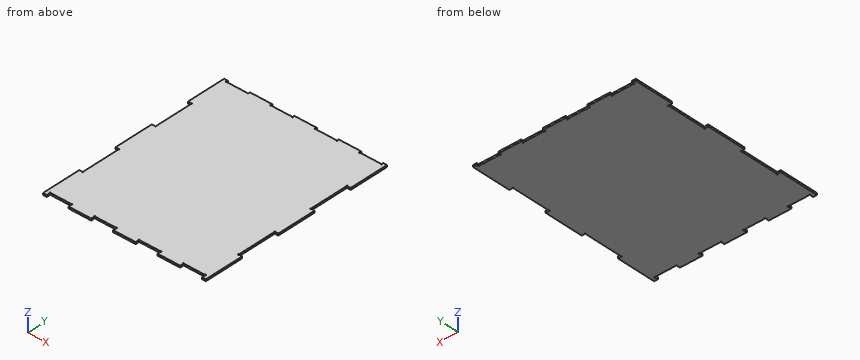
Autodesk Inventor part; units mm, degrees
ref_plane "YZ Plane" through (0, 0, 0) normal (1, 0, 0) x (0, 1, 0)
ref_plane "XZ Plane" through (0, 0, 0) normal (0, 1, 0) x (-1, 0, 0)
ref_plane "XY Plane" through (0, 0, 0) normal (0, 0, 1) x (1, 0, 0)
sketch "Esboço1" plane through (0, 0, 0) normal (0, 0, 1) x (1, 0, 0)
  line L0 (-173, 210) -> (173, 210)
  line L1 (173, 210) -> (173, -210)
  line L2 (173, -210) -> (-173, -210)
  line L3 (-173, -210) -> (-173, 210)
  point P0 (0, 0)
  point P1 (173, 0)
  point P2 (0, 210)
  dimension "d0" = 420
  dimension "d1" = 346
extrude "Extrusão1" add sketch "Esboço1" along normal blind 4
sketch "Esboço2" plane through (0, 0, 4) normal (0, 0, 1) x (1, 0, 0)
  line L0 (-173, 210) -> (-173, -210)
  line L1 (-173, -210) -> (173, -210)
  line L2 (-165, -202) -> (-118.5, -202)
  line L3 (-118.5, -202) -> (-118.5, -210)
  line L4 (-118.5, -210) -> (-165, -210)
  line L5 (-70.5, -210) -> (-24, -210)
  line L6 (-24, -210) -> (-24, -202)
  line L7 (-24, -202) -> (-70.5, -202)
  line L8 (-70.5, -202) -> (-70.5, -210)
  line L9 (24, -210) -> (70.5, -210)
  line L10 (70.5, -210) -> (70.5, -202)
  line L11 (70.5, -202) -> (24, -202)
  line L12 (24, -202) -> (24, -210)
  line L13 (118.5, -210) -> (165, -210)
  line L14 (165, -210) -> (165, -202)
  line L15 (165, -202) -> (118.5, -202)
  line L16 (118.5, -202) -> (118.5, -210)
  circle A0 centre (-118.5, -202) radius 1
  circle A1 centre (-70.5, -202) radius 1
  circle A2 centre (-24, -202) radius 1
  circle A3 centre (24, -202) radius 1
  circle A4 centre (70.5, -202) radius 1
  circle A5 centre (118.5, -202) radius 1
  line L17 (173, -210) -> (173, 210)
  line L18 (-165, -202) -> (-165, -210)
  circle A6 centre (165, -202) radius 1
  circle A7 centre (-165, -202) radius 1
  point P0 (0, 0)
  dimension "d4" = 46.5
  dimension "d5" = 8
  dimension "d6" = 46.5
  dimension "d7" = 46.5
  dimension "d8" = 46.5
  dimension "d9" = 8
  dimension "d10" = 8
  dimension "d11" = 48
  dimension "d12" = 48
  dimension "d13" = 48
  dimension "d16" = 2
  dimension "d17" = 2
  dimension "d18" = 2
  dimension "d19" = 2
  dimension "d20" = 2
  dimension "d21" = 2
  dimension "d38" = 8
  dimension "d40" = 46.5
  dimension "d41" = 2
  dimension "d42" = 2
extrude "Extrusão2" cut sketch "Esboço2" against normal blind 10
sketch "Esboço3" plane through (0, 0, 0) normal (0, 0, -1) x (-1, 0, 0)
  line L0 (-173, 210) -> (173, 210)
  line L1 (-118.5, 210) -> (-118.5, 206)
  line L2 (-118.5, 206) -> (-165, 206)
  line L3 (-70.5, 210) -> (-24, 210)
  line L4 (-24, 210) -> (-24, 206)
  line L5 (-24, 206) -> (-70.5, 206)
  line L6 (-70.5, 206) -> (-70.5, 210)
  line L7 (173, -210) -> (173, 210)
  circle A0 centre (-118.5, 206) radius 1
  circle A1 centre (-70.5, 206) radius 1
  circle A2 centre (-24, 206) radius 1
  line L8 (-165, 206) -> (-165, 210)
  line L9 (-118.5, 210) -> (-165, 210)
  line L10 (173, 210) -> (-173, 210)
  line L11 (-173, 210) -> (-173, -210)
  circle A3 centre (-165, 206) radius 1
  point P0 (0, 0)
  point P1 (173, -202)
  dimension "d22" = 46.5
  dimension "d23" = 4
  dimension "d24" = 46.5
  dimension "d31" = 48
  dimension "d33" = 2
  dimension "d34" = 2
  dimension "d35" = 2
  dimension "d43" = 8
  dimension "d44" = 2
extrude "Extrusão3" cut sketch "Esboço3" against normal blind 10
mirror "Espelhamento1" about plane through (0, 0, 0) normal (1, 0, 0) of "Extrusão3"
sketch "Esboço4" plane through (0, 0, 0) normal (0, 0, -1) x (-1, 0, 0)
  line L0 (173.5526, -126) -> (165.5526, -126)
  line L1 (165.5526, -126) -> (165.5526, -42)
  line L2 (165.5526, -42) -> (173.5526, -42)
  line L3 (173.5526, -42) -> (173.5526, -126)
  line L4 (165, -210) -> (173, -210)
  line L5 (173, 210) -> (173, -210)
  line L6 (173, 42) -> (165, 42)
  line L7 (165, 42) -> (165, 126)
  line L8 (165, 126) -> (173, 126)
  line L9 (173, 126) -> (173, 42)
  line L10 (173, 210) -> (165, 210)
  circle A0 centre (165.5526, -42) radius 1
  circle A1 centre (165.5526, -126) radius 1
  circle A2 centre (165, 42) radius 1
  circle A3 centre (165, 126) radius 1
  point P0 (0, 0)
  dimension "d45" = 8
  dimension "d46" = 84
  dimension "d47" = 84
  dimension "d48" = 84
  dimension "d49" = 84
  dimension "d50" = 84
  dimension "d51" = 2
  dimension "d52" = 2
  dimension "d53" = 2
  dimension "d54" = 2
extrude "Extrusão4" cut sketch "Esboço4" against normal blind 10
mirror "Espelhamento2" about plane through (0, 0, 0) normal (1, 0, 0) of "Extrusão4"
properties part number "traseira"
Input: part model. Units: mm. Frame: model coordinates. Coordinates: 2 decimals unless noted, no trailing zeros. Order: outer loops, then holes, each group sorted by start corner. A loop starts at its lowest first (then second) coordinate and runs counter-clockwise, first axis right, second up. Notation, with made-up numbers: M -12.75,42.25 L 0.25,42.25 A20 ccw 0.25,70.25 Z; hole C -34.75,75 d6. An arc over 180 degrees is marked long. Answer in a Markdown table with one row per item.
(1) Contact query for flat-ended pins moving along their axis: pin 1 Ø2 at (y, z) = (51, 0.5) entering from +X; pin 2 Ø2 at (y, z) = (-80, 1.5) entering from -X; pin 3 Ø1.2 at (x, y) = (-165, -202) entering from +Z; pin 4 Ø1.2 at (x, z) = (-50.5, 1.5) entering from +Y. Output: stop coordinate, or through.
Numbers:
| item | result |
|---|---|
| pin 1 | stops at x = 165 |
| pin 2 | stops at x = -165.55 |
| pin 3 | passes through |
| pin 4 | stops at y = 206 |
(2) Section query B-B, the plane x = 60.5. Output: boundary loops of the cut face in (y, z).
Numbers:
| item | result |
|---|---|
| outline | M -202,0 L 206,0 L 206,4 L -202,4 Z |
(3) Material intervals for line 1 (Y direction, x = 130, z = 0.6); line 2 (X direction, y = -109, z = 3.25); line 3 (X direction, y = 46, z = 1.8), sorted ascending. Write a range as [from, to].
Numbers:
| item | result |
|---|---|
| line 1 | y = [-202, 206] |
| line 2 | x = [-165.55, 165.55] |
| line 3 | x = [-165, 165] |
(4) Section query A-A, the plane y = 102.5. Output: boundary loops of the cut face in (x, z), plus the area to 3 significant figures.
Numbers:
| item | result |
|---|---|
| outline | M -165,0 L 165,0 L 165,4 L -165,4 Z |
| area | 1,320 mm^2 |
